from build123d import *

# Parameters (mm, degrees)
F0_R     = 13.9
F0_R_2   = 12.4
F1_DEPTH = 10
F0_R_3   = 9.3
F2_DEPTH = 9
F0_R_4   = 5.1
F3_DEPTH = 20
F4_SIZE  = 0.5
F5_SIZE  = 0.99999


# Not quite as in the source:
# - a fillet or chamfer is up to 0.001 mm smaller than in the source, because OpenCascade refuses the exact size


with BuildPart() as f1:
    # F0 (on Top) → F1 (new body)
    with BuildSketch(Plane.XY):
        Circle(F0_R)
        Circle(F0_R_2, mode=Mode.SUBTRACT)
    extrude(amount=F1_DEPTH)

    # F0 (on Top) → F2 (join)
    with BuildSketch(Plane.XY):
        Circle(F0_R)
        Circle(F0_R_2, mode=Mode.SUBTRACT)
        Circle(F0_R_2)
        Circle(F0_R_3, mode=Mode.SUBTRACT)
    extrude(amount=F2_DEPTH)

    # F0 (on Top) → F3 (join)
    with BuildSketch(Plane.XY):
        Circle(F0_R_3)
        Circle(F0_R_4, mode=Mode.SUBTRACT)
    extrude(amount=F3_DEPTH)

    # F4
    f4_edges = [f1.edges().sort_by_distance(p)[0] for p in [
        (-5.1, 0, 20),
        (-9.3, 0, 20),
        (-9.3, 0, 9),
        (-5.1, 0, 0),
    ]]
    chamfer(f4_edges, length=F4_SIZE)

    # F5 (size 1 in the source; OpenCascade refuses exactly that, so slightly less here)
    f5_edges = [f1.edges().sort_by_distance(p)[0] for p in [
        (-12.4, 0, 9),
    ]]
    chamfer(f5_edges, length=F5_SIZE)


solid = f1.part
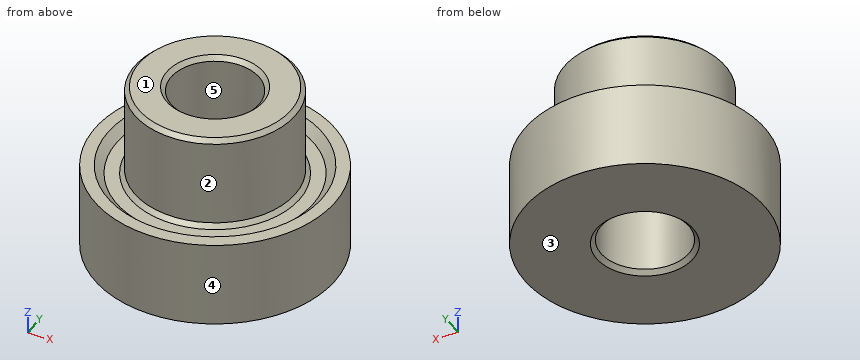
Design review of the part built by this model. Coordinates are the model's own, in mm. Face numbers are marked on the shaded views. A direction names the side the tool comes from. Round coordinates to 2 decimals unless told otherwise and drop trailing zeros. Loops run counter-clockwise (first coordinate to the right, second up) from the corner with the lowest first, then second, coordinate; pieces in that order, holes last. Notation, with made-up numbers: (-40, 76.5) - (-5, 76.5) arc R14 ccw to (-5, 83.5) - close; hole circle Ø7 at (28, 26). An arc over 180 degrees is marked (long way). One line per question, with ' | ' between items.
1. We need section C-C, the plane z = 14.75. State the section outline as (x, y) points, and give its area (3 significant figures).
Results are:
outline: circle Ø18.6 at (0, 0); hole circle Ø10.2 at (0, 0) | area: 190 mm²
2. Draft analysis for pull direction X (two halves, no side actions). For the marked faces 3, 4 and 5, state which applies: released by +X, released by -X, zero draft, split by the parting line, or undercut.
Results are:
face 3: zero draft | face 4: split by the parting line | face 5: undercut
3. We need section D-D, the plane z = 8.25. State the section outline as (x, y) points, and give its area (3 significant figures).
Results are:
outline: circle Ø27.8 at (0, 0); hole circle Ø10.2 at (0, 0) | area: 525 mm²
4. For L1, parallel to Y at x = 0, z = 6.75; L2, parallel to Y at x = 0, z = 10.05; L3, parallel to Z at x = 5.5, y = -1, list the stretches that pass through material, from the lowest coordinate up. Write a range as [from, to].
Results are:
L1: y = [-13.9, -5.1], [5.1, 13.9] | L2: y = [-9.3, -5.1], [5.1, 9.3] | L3: z = [0.01, 19.99]
5. For the marked faces 1 and 2, list the 3-axis set-ups (+Z, -Z, +X, -X, +Y, -Y) from which the entire face can be reached by the end or side of a thin tool; tool diameter is ignored.
Results are:
face 1: +Z, +X, -X, +Y, -Y | face 2: +Z
6. Clearance check with flat-ended pins moving along their axes: P1, Ø3, axis at x = -7, z = 3.5, coming from the -Y side; P2, Ø6, axis at x = 9.5, z = 17, coming from the -Y side; P3, Ø1, axis at y = 3.5, z = 15.5, coming from the -X side. State where each tip first meets the part, or that it passes through.
Results are:
P1: stops at y = -12.77 | P2: stops at y = -6.65 | P3: stops at x = -8.8
